Geometry check sheet. Reference: the model listing, model coordinates, mm. Coordinates: 2 decimals unless noted, no trailing zeros. Write each loop counter-clockwise with the first axis right and the second up, starting at its lowest first coordinate (ties: lowest second). Pieces come first, ordered by that corner, then holes. Notation, with made-up numbers: (52.5, 83.5) -> (65.5, 83.5) arc R18 cw to (65.5, 115.5) -> close; hole circle Ø7 at (82, -17.5). An arc over 180 degrees is marked (long way). Answer in a Markdown table with one row per item. Add a question column.
1. Cross-section at A-A on y = -0.5. Record the cut outline in (x, z).
2. Cross-section at C-C on z = 133.5. Record the cut outline in (x, y), and give its area (3 significant figures).
3. Cross-section at B-B on x = 149.5. Record the cut outline in (y, z), and give its area (3 significant figures).
4. Scan lines: L1, parallel to X at y = -0.5, z = -121; L2, parallel to Z at x = -126, y = -0.4. Record each from-to range of solid material in increasing order. Write a range as from..to.
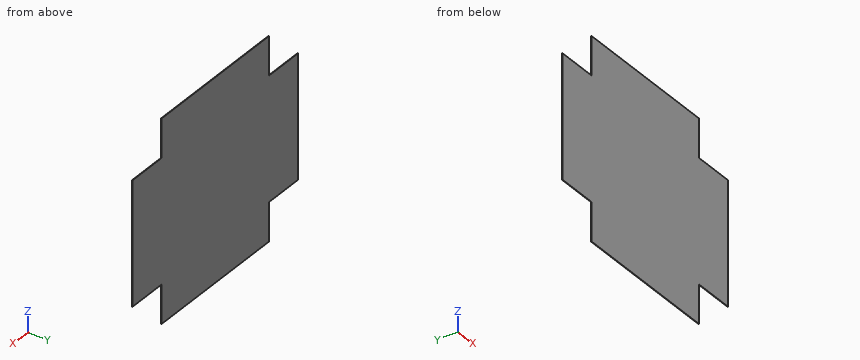
```python
from build123d import *

# Parameters (mm, degrees)
BASE_FLANGE1_DEPTH = 0.7366


# Sheet-metal steps are written as plain solids
with BuildPart() as part:
    # Sketch1 → Base-Flange1 (new body)
    with BuildSketch(Plane(origin=(0, 0, 0), x_dir=(1, 0, 0), z_dir=(0, 1, 0))):
        Polygon((-127, 101.6), (-123.25, 101.6), (-123.25, 165.1), (123.25, 165.1), (123.25, 101.6), (127, 101.6), (190.5, 101.6), (190.5, -101.6), (127, -101.6), (123.25, -101.6), (123.25, -165.1), (-123.25, -165.1), (-123.25, -101.6), (-127, -101.6), (-190.5, -101.6), (-190.5, 101.6), align=None)
    extrude(amount=-BASE_FLANGE1_DEPTH)


solid = part.part
```
Results found:
| question | item | result |
|---|---|---|
| 1 | outline | (-190.5, -101.6) -> (-123.25, -101.6) -> (-123.25, -165.1) -> (123.25, -165.1) -> (123.25, -101.6) -> (190.5, -101.6) -> (190.5, 101.6) -> (123.25, 101.6) -> (123.25, 165.1) -> (-123.25, 165.1) -> (-123.25, 101.6) -> (-190.5, 101.6) -> close |
| 2 | outline | (-123.25, -0.74) -> (123.25, -0.74) -> (123.25, 0) -> (-123.25, 0) -> close |
| 2 | area | 182 mm^2 |
| 3 | outline | (-0.74, -101.6) -> (0, -101.6) -> (0, 101.6) -> (-0.74, 101.6) -> close |
| 3 | area | 150 mm^2 |
| 4 | L1 | x = -123.25..123.25 |
| 4 | L2 | z = -101.6..101.6 |
